Autodesk Inventor part; units mm, degrees
ref_plane "Work Plane1" through (-2.7515, 150, 3.6) normal (0, 1, 0) x (1, 0, 0)
ref_plane "YZ Plane" through (0, 0, 0) normal (1, 0, 0) x (0, 1, 0)
ref_plane "XZ Plane" through (0, 0, 0) normal (0, 1, 0) x (-1, 0, 0)
ref_plane "Work Plane1" through (-2.7515, 150, 3.6) normal (0, 1, 0) x (1, 0, 0)
sketch "Sketch1" plane through (-2.7515, 150, 3.6) normal (0, 1, 0) x (1, 0, 0)
  arc A0 (-6.7485, 13.6) -> (-7.2485, 13.1) centre (-6.7485, 13.1) ccw
  line L0 (-7.2485, 13.1) -> (-7.2485, 8.1)
  line L1 (-7.2485, 8.1) -> (-5.7485, 6.6)
  line L2 (-5.7485, 6.6) -> (-5.7485, 9.8)
  line L3 (-5.7485, 9.8) -> (-4.2971, 9.8)
  line L4 (-4.2971, 9.8) -> (-0.8485, 6.3515)
  line L5 (-0.8485, 6.3515) -> (-0.8485, 0.8485)
  line L6 (-0.8485, 0.8485) -> (-4.2971, -2.6)
  line L7 (-4.2971, -2.6) -> (-5.7485, -2.6)
  line L8 (-5.7485, -2.6) -> (-5.7485, 0.6)
  line L9 (-5.7485, 0.6) -> (-7.2485, -0.9)
  line L10 (-7.2485, -0.9) -> (-7.2485, -5.9)
  arc A1 (-7.2485, -5.9) -> (-6.7485, -6.4) centre (-6.7485, -5.9) ccw
  line L11 (-6.7485, -6.4) -> (-1.7485, -6.4)
  line L12 (-1.7485, -6.4) -> (-0.2485, -4.9)
  line L13 (-0.2485, -4.9) -> (-3.4485, -4.9)
  line L14 (-3.4485, -4.9) -> (-3.4485, -3.4485)
  line L15 (-3.4485, -3.4485) -> (0, 0)
  line L16 (0, 0) -> (5.5029, 0)
  line L17 (5.5029, 0) -> (8.9515, -3.4485)
  line L18 (8.9515, -3.4485) -> (8.9515, -4.9)
  line L19 (8.9515, -4.9) -> (5.7515, -4.9)
  line L20 (5.7515, -4.9) -> (7.2515, -6.4)
  line L21 (7.2515, -6.4) -> (12.2515, -6.4)
  arc A2 (12.2515, -6.4) -> (12.7515, -5.9) centre (12.2515, -5.9) ccw
  line L22 (12.7515, -5.9) -> (12.7515, -0.9)
  line L23 (12.7515, -0.9) -> (11.2515, 0.6)
  line L24 (11.2515, 0.6) -> (11.2515, -2.6)
  line L25 (11.2515, -2.6) -> (9.8, -2.6)
  line L26 (9.8, -2.6) -> (6.3515, 0.8485)
  line L27 (6.3515, 0.8485) -> (6.3515, 6.3515)
  line L28 (6.3515, 6.3515) -> (9.8, 9.8)
  line L29 (9.8, 9.8) -> (11.2515, 9.8)
  line L30 (11.2515, 9.8) -> (11.2515, 6.6)
  line L31 (11.2515, 6.6) -> (12.7515, 8.1)
  line L32 (12.7515, 8.1) -> (12.7515, 13.1)
  arc A3 (12.7515, 13.1) -> (12.2515, 13.6) centre (12.2515, 13.1) ccw
  line L33 (12.2515, 13.6) -> (7.2515, 13.6)
  line L34 (7.2515, 13.6) -> (5.7515, 12.1)
  line L35 (5.7515, 12.1) -> (8.9515, 12.1)
  line L36 (8.9515, 12.1) -> (8.9515, 10.6485)
  line L37 (8.9515, 10.6485) -> (5.5029, 7.2)
  line L38 (5.5029, 7.2) -> (0, 7.2)
  line L39 (0, 7.2) -> (-3.4485, 10.6485)
  line L40 (-3.4485, 10.6485) -> (-3.4485, 12.1)
  line L41 (-3.4485, 12.1) -> (-0.2485, 12.1)
  line L42 (-0.2485, 12.1) -> (-1.7485, 13.6)
  line L43 (-1.7485, 13.6) -> (-6.7485, 13.6)
  circle A4 centre (2.7515, 3.6) radius 2
extrude "Extrusion1" add sketch "Sketch1" along normal blind 330
ref_plane "Work Plane2" through (0, 150, -9.5) normal (1, 0, 0) x (0, 0, -1)
ref_plane "Work Plane3" through (-4.5, 150, 0) normal (0, 0, 1) x (1, 0, 0)
properties part number "20x20mmx150mm alminum profile" material "Aluminum 6061"
The listing builds one solid part. Answer for the finished solid, in the listing's coordinates (mm). A direction names the side the tool comes from. Coordinates: 2 decimals unless noted, no trailing zeros. Return JSON: item names as keys, results as strings. Group by question number.
Q1. Find the intervals of material crossed by line 1 along Z through (x, y) = (0, 407.5); line 2 along X through (y, z) = (280, -5), in increasing order. Write a range as [from, to].
Q2. For a pull along Z with two mould halves and no side action, classify faces 1 (the flat face through (3.6, 313, 0)), 2 (the flat face through (0, 313, 3.6)), 3 (the flat face through (7, 313, -10)) as +Z half, -Z half, draft (parallel to the pull), parting line (faces both ways), or undercut.
Q3. Flat-ended cylindrical pins translate along their axes: pin 1 Ø4 at (y, z) = (422, 2) entering from -X; pin 2 Ø6 at (x, y) = (-1, 288) entering from -Z. Find the tip coordinate at first contact, or state that the pin passes through.
Q4. Which of the six approach directions +Z, -Z, +X, -X, +Y, -Y give full straight-line access (tool end or side, diameter ignored) to faces 4 (the flat face through (0, 313, -3.6)), 5 (the flat face through (-3.6, 313, 0)), 6 (the flat face through (10, 313, -7))?
Evaluation:
{
 "1": {"line 1": "z = [-3.6, -2], [2, 3.6]", "line 2": "x = [-10, -8.5], [-5.85, -4.15], [4.15, 5.85], [8.5, 10]"},
 "2": {"face 1": "undercut", "face 2": "+Z half", "face 3": "-Z half"},
 "3": {"pin 1": "stops at x = -9.5", "pin 2": "stops at z = -9.5"},
 "4": {"face 4": "-Z, +Y, -Y", "face 5": "-X, +Y, -Y", "face 6": "+Z, -Z, +X, +Y, -Y"}
}
